Verification items for the finished model (mm, model axes). A direction names the side the tool comes from. Round coordinates to 2 decimals unless told otherwise and drop trailing zeros. Write each loop counter-clockwise with the first axis right and the second up, starting at its lowest first coordinate (ties: lowest second). Pieces come first, ordered by that corner, then holes. Notation, with made-up numbers: (-5.5, 66.5) - (-0.5, 66.5) arc R18 cw to (-0.5, 88.5) - close; hole circle Ø6 at (77.25, 9). An arc over 180 degrees is marked (long way). Answer as a JSON object with one key per item and string values. Group by question number.
1) Mould release check, pull along X, two halves, no side actions. Record for faces 3 (the flat face through (-3.5, 0, 294)), 4 (the flat face through (5, 0, 294)), 5 (the flat face through (-5, 0, 294)), 6 (the flat face through (-4.5, 0.1, 0)): +X half, -X half, draft (parallel to the pull), parting line (faces both ways), or undercut.
2) Go/stop test with a flat-tipped pin: pin 1 Ø6.5 at (y, z) = (0, 250) entering from -X. Record where the tip stops, or that it passes through.
3) Section check B-B (z = 502.5). Enter the section's corners in (x, y).
4) Section check A-A (x = -1.75). Enter the section's corners in (y, z).
5) Thickness scan on line 1 (Y direction, x = 4.55, z = 591); line 2 (Y direction, x = -2, z = 534); line 3 (X direction, y = -5, z = 425). Record the ranges inside material, lowest first.
6) Set-up check for faces 1 (the flat face through (3.5, 0, 294)), 2 (the flat face through (0, -7.5, 294)): record each of +Z, -Z, +X, -X, +Y, -Y from which the full face is reachable in a straight line by a thin tool's end or side.
```python
from build123d import *

# Parameters (mm, degrees)
SKETCH_1_W          = 10
SKETCH_1_H          = 15
SKETCH_1_W_2        = 7
SKETCH_1_H_2        = 12
EXTRUDE_1_DEPTH     = 596
SKETCH_2_R          = 1.5
SKETCH_2_R_2        = 2.5
SKETCH_2_R_3        = 2
CUT_EXTRUDE_1_DEPTH = 597.131067803
SKETCH_3_R          = 4
CUT_EXTRUDE_2_DEPTH = 1.5


with BuildPart() as part:
    # ｽｹｯﾁ1 → 押し出し-薄板1 (new body)
    with BuildSketch(Plane.XY):
        Rectangle(SKETCH_1_W, SKETCH_1_H)
        Rectangle(SKETCH_1_W_2, SKETCH_1_H_2, mode=Mode.SUBTRACT)
    extrude(amount=EXTRUDE_1_DEPTH)

    # ｽｹｯﾁ2 → ｶｯﾄ - 押し出し1 (cut, through all)
    with BuildSketch(Plane(origin=(5, 0, 0), x_dir=(0, 0, -1), z_dir=(1, 0, 0))):
        with Locations((-5, 4)):
            Circle(SKETCH_2_R)
        with Locations((-5, -4)):
            Circle(SKETCH_2_R)
        with Locations((-591, 4)):
            Circle(SKETCH_2_R)
        with Locations((-591, -4)):
            Circle(SKETCH_2_R)
        with Locations((-50, 0)):
            Circle(SKETCH_2_R_2)
        with Locations((-567, 0)):
            Circle(SKETCH_2_R)
        with Locations((-530, 0)):
            Circle(SKETCH_2_R_2)
        with Locations((-250, 0)):
            Circle(SKETCH_2_R_3)
        with Locations((-270, 0)):
            Circle(SKETCH_2_R_3)
        with Locations((-450, 0)):
            Circle(SKETCH_2_R_2)
        with Locations((-290, 0)):
            Circle(SKETCH_2_R_2)
        with Locations((-210, 0)):
            Circle(SKETCH_2_R_2)
        with Locations((-130, 0)):
            Circle(SKETCH_2_R_2)
    extrude(amount=-CUT_EXTRUDE_1_DEPTH, mode=Mode.SUBTRACT)

    # ｽｹｯﾁ3 → ｶｯﾄ - 押し出し2 (cut)
    with BuildSketch(Plane.ZY.offset(5)):
        with Locations((250, 0)):
            Circle(SKETCH_3_R)
        with Locations((270, 0)):
            Circle(SKETCH_3_R)
    extrude(amount=-CUT_EXTRUDE_2_DEPTH, mode=Mode.SUBTRACT)


solid = part.part
```
Returned:
{
 "1": {"face 3": "undercut", "face 4": "+X half", "face 5": "-X half", "face 6": "draft"},
 "2": {"pin 1": "x = 3.5"},
 "3": {"outline": "(-5, -7.5) - (5, -7.5) - (5, 7.5) - (-5, 7.5) - close; hole (-3.5, -6) - (3.5, -6) - (3.5, 6) - (-3.5, 6) - close"},
 "4": {"outline": "(-7.5, 0) - (-6, 0) - (-6, 596) - (-7.5, 596) - close; (6, 0) - (7.5, 0) - (7.5, 596) - (6, 596) - close"},
 "5": {"line 1": "-7.5 to -5.5, -2.5 to 2.5, 5.5 to 7.5", "line 2": "-7.5 to -6, 6 to 7.5", "line 3": "-5 to -3.5, 3.5 to 5"},
 "6": {"face 1": "+Z, -Z", "face 2": "+Z, -Z, +X, -X, -Y"}
}
